For this review, take the finished solid that the model builds, in its own axes (mm). A direction names the side the tool comes from. Round coordinates to 2 decimals unless told otherwise and drop trailing zeros. Write each loop counter-clockwise with the first axis right and the second up, starting at its lowest first coordinate (ties: lowest second). Pieces come first, ordered by that corner, then holes.
from build123d import *

# Parameters (mm, degrees)
CYLINDER004_R             = 1.75
CYLINDER004_DEPTH         = 30
BOX005_W                  = 20
BOX005_H                  = 6
BOX005_DEPTH              = 3
PRISM004_DEPTH            = 3
FUSION004_PLACEMENT_ANGLE = 180
CYLINDER003_R             = 1.75
CYLINDER003_DEPTH         = 30
BOX004_W                  = 20
BOX004_H                  = 6
BOX004_DEPTH              = 3
PRISM003_DEPTH            = 3
FUSION003_PLACEMENT_ANGLE = 180
CYLINDER002_R             = 1.75
CYLINDER002_DEPTH         = 30
BOX003_W                  = 20
BOX003_H                  = 6
BOX003_DEPTH              = 3
PRISM002_DEPTH            = 3
CYLINDER001_R             = 1.75
CYLINDER001_DEPTH         = 30
BOX002_W                  = 20
BOX002_H                  = 6
BOX002_DEPTH              = 3
PRISM001_DEPTH            = 3
BOX_W                     = 40
BOX_H                     = 46
BOX_DEPTH                 = 7
PAD_DEPTH                 = 4


with BuildPart() as cilindro004:
    # Cylinder004 → Cylinder004 (new body)
    with BuildSketch(Plane.XY.offset(-5)):
        Circle(CYLINDER004_R)
    extrude(amount=CYLINDER004_DEPTH)


with BuildPart() as cubo005:
    # Box005 → Box005 (new body)
    with BuildSketch(Plane(origin=(1, -3, 0), x_dir=(1, 0, 0), z_dir=(0, 0, 1))):
        with Locations((10, 3)):
            Rectangle(BOX005_W, BOX005_H)
    extrude(amount=BOX005_DEPTH)


with BuildPart() as fusion004:
    # Prism004 → Prism004 (new body)
    with BuildSketch(Plane.XY):
        Polygon((3.25, 0), (1.625, 2.814583), (-1.625, 2.814583), (-3.25, 0), (-1.625, -2.814583), (1.625, -2.814583), align=None)
    extrude(amount=PRISM004_DEPTH)

    # Fusion004: union Cilindro004, Cubo005
    add(cilindro004.part)
    add(cubo005.part)


with BuildPart() as fusion004_1:
    # Fusion004 placement: moved
    add(fusion004.part.moved(Location((5, 35, 2))).rotate(Axis((5, 35, 2), (0, 0, 1)), FUSION004_PLACEMENT_ANGLE))


with BuildPart() as cilindro003:
    # Cylinder003 → Cylinder003 (new body)
    with BuildSketch(Plane.XY.offset(-5)):
        Circle(CYLINDER003_R)
    extrude(amount=CYLINDER003_DEPTH)


with BuildPart() as cubo004:
    # Box004 → Box004 (new body)
    with BuildSketch(Plane(origin=(1, -3, 0), x_dir=(1, 0, 0), z_dir=(0, 0, 1))):
        with Locations((10, 3)):
            Rectangle(BOX004_W, BOX004_H)
    extrude(amount=BOX004_DEPTH)


with BuildPart() as fusion003:
    # Prism003 → Prism003 (new body)
    with BuildSketch(Plane.XY):
        Polygon((3.25, 0), (1.625, 2.814583), (-1.625, 2.814583), (-3.25, 0), (-1.625, -2.814583), (1.625, -2.814583), align=None)
    extrude(amount=PRISM003_DEPTH)

    # Fusion003: union Cilindro003, Cubo004
    add(cilindro003.part)
    add(cubo004.part)


with BuildPart() as fusion003_1:
    # Fusion003 placement: moved
    add(fusion003.part.moved(Location((5, 5, 2))).rotate(Axis((5, 5, 2), (0, 0, 1)), FUSION003_PLACEMENT_ANGLE))


with BuildPart() as cilindro002:
    # Cylinder002 → Cylinder002 (new body)
    with BuildSketch(Plane.XY.offset(-5)):
        Circle(CYLINDER002_R)
    extrude(amount=CYLINDER002_DEPTH)


with BuildPart() as cubo003:
    # Box003 → Box003 (new body)
    with BuildSketch(Plane(origin=(1, -3, 0), x_dir=(1, 0, 0), z_dir=(0, 0, 1))):
        with Locations((10, 3)):
            Rectangle(BOX003_W, BOX003_H)
    extrude(amount=BOX003_DEPTH)


with BuildPart() as fusion002:
    # Prism002 → Prism002 (new body)
    with BuildSketch(Plane.XY):
        Polygon((3.25, 0), (1.625, 2.814583), (-1.625, 2.814583), (-3.25, 0), (-1.625, -2.814583), (1.625, -2.814583), align=None)
    extrude(amount=PRISM002_DEPTH)

    # Fusion002: union Cilindro002, Cubo003
    add(cilindro002.part)
    add(cubo003.part)


with BuildPart() as fusion002_1:
    # Fusion002 placement: moved
    add(fusion002.part.moved(Location((35, 35, 2))))


with BuildPart() as cilindro001:
    # Cylinder001 → Cylinder001 (new body)
    with BuildSketch(Plane.XY.offset(-5)):
        Circle(CYLINDER001_R)
    extrude(amount=CYLINDER001_DEPTH)


with BuildPart() as cubo002:
    # Box002 → Box002 (new body)
    with BuildSketch(Plane(origin=(1, -3, 0), x_dir=(1, 0, 0), z_dir=(0, 0, 1))):
        with Locations((10, 3)):
            Rectangle(BOX002_W, BOX002_H)
    extrude(amount=BOX002_DEPTH)


with BuildPart() as fusion001:
    # Prism001 → Prism001 (new body)
    with BuildSketch(Plane.XY):
        Polygon((3.25, 0), (1.625, 2.814583), (-1.625, 2.814583), (-3.25, 0), (-1.625, -2.814583), (1.625, -2.814583), align=None)
    extrude(amount=PRISM001_DEPTH)

    # Fusion001: union Cilindro001, Cubo002
    add(cilindro001.part)
    add(cubo002.part)


with BuildPart() as fusion001_1:
    # Fusion001 placement: moved
    add(fusion001.part.moved(Location((35, 5, 2))))


with BuildPart() as body:
    # Box → Box (new body)
    with BuildSketch(Plane.XY):
        with Locations((20, 23)):
            Rectangle(BOX_W, BOX_H)
    extrude(amount=BOX_DEPTH)

    # Cut: cut Fusion001
    add(fusion001_1.part, mode=Mode.SUBTRACT)

    # Cut001: cut Fusion002
    add(fusion002_1.part, mode=Mode.SUBTRACT)

    # Cut002: cut Fusion003
    add(fusion003_1.part, mode=Mode.SUBTRACT)

    # Cut003: cut Fusion004
    add(fusion004_1.part, mode=Mode.SUBTRACT)

    # Sketch → Pad (new body)
    with BuildSketch(Plane.XZ):
        with BuildLine():
            Line((0, 0), (10, 0))
            ThreePointArc((30, -2.8e-05), (20.000014, 9.999972), (10, 0))
            Line((30, -2.8e-05), (40, -2.8e-05))
            ThreePointArc((40, -2.8e-05), (20.000014, 19.999972), (0, 0))
        make_face()
        with BuildLine():
            ThreePointArc((37, 1), (20, 17.02936), (3, 1))
            Line((3, 1), (7, 1))
            ThreePointArc((33, 1), (20, 13.038379), (7, 1))
            Line((37, 1), (33, 1))
        make_face(mode=Mode.SUBTRACT)
    extrude(amount=PAD_DEPTH)


solid = body.part
(1) We need section C-C, the plane y = 22.5. Give the boundary of the cut face in (x, z), and give its area (3 significant figures).
Geometry check:
outline: (0, 0) - (40, 0) - (40, 7) - (0, 7) - close
area: 280 mm2
(2) For line 1 along Y through (x, z) = (5, 0.6); line 2 along Y through (x, z) = (5, 6.1); line 3 along Z through (x, y) = (37, 19), list the stretches that pass through material, from the lowest coordinate up.
Geometry check:
line 1: y = -4 to 3.25, 6.75 to 33.25, 36.75 to 46
line 2: y = 0 to 3.25, 6.75 to 33.25, 36.75 to 46
line 3: z = 0 to 7
(3) We need section B-B, the plane x = 29. Give the boundary of the cut face in (y, z).
Geometry check:
outline: (-4, 4.36) - (0, 4.36) - (0, 0) - (46, 0) - (46, 7) - (0, 7) - (0, 9.43) - (-4, 9.43) - close; (-4, 14.46) - (0, 14.46) - (0, 17.86) - (-4, 17.86) - close
(4) For faces 1 (the face through (37, 4, 2)), 2 (the face through (35, 0, 4)), 3 (the face through (20, -2, 20)), 4 (the face through (7.426, 33.573, 3.479)), 5 (the face through (0.4, 0, 5.3)), list the 3-axis set-ups (+Z, -Z, +X, -X, +Y, -Y) from which the entire face can be reached by the end or side of a thin tool; tool diameter is ignored.
Geometry check:
face 1: +X
face 2: -Y
face 3: +Z, -Y
face 4: -X
face 5: +Z, -X, -Y
(5) Mouldability with a two-part tool opening along Z and no side actions: class faces 6 (the face through (20, 23, 7)), 7 (the face through (32.551, 3.612, 3.479)), 8 (the face through (0, 23, 3)) as pulls with the +Z half, pulls with the -Z half, needs draft (parallel to the pull), parting line crosses it, or undercut.
Geometry check:
face 6: pulls with the +Z half
face 7: undercut
face 8: needs draft
(6) For pin 1 Ø2 at (x, z) = (5, 3) entering from -Y; pin 2 Ø3 at (x, y) = (9.5, 39) entering from +Z; pin 3 Ø2 at (x, y) = (35, -2) entering from +Z, all flat-tipped, find the tip position at first contact; note any pin that passes through.
Geometry check:
pin 1: stops at y = 0
pin 2: stops at z = 7
pin 3: stops at z = 14.28
(7) We need section D-D, the plane z = 18.5. Give the boundary of the cut face in (x, y), and give its area (3 significant figures).
Geometry check:
outline: (12.4, -4) - (27.6, -4) - (27.6, 0) - (12.4, 0) - close
area: 60.8 mm2
(8) We need section A-A, the plane x = 20. Give the boundary of the cut face in (y, z), and give its area (3 significant figures).
Geometry check:
outline: (-4, 10) - (0, 10) - (0, 13.04) - (-4, 13.04) - close; (-4, 17.03) - (0, 17.03) - (0, 20) - (-4, 20) - close; (0, 0) - (46, 0) - (46, 7) - (0, 7) - close
area: 346 mm2
